Part model, mm, in its own coordinate system. A direction names the side the tool comes from. Round coordinates to 2 decimals unless told otherwise and drop trailing zeros. Loops run counter-clockwise (first coordinate to the right, second up) from the corner with the lowest first, then second, coordinate; pieces in that order, holes last.
(1) Tool access for faces 1 (the face through (48.6, 100.5, -4)), 2 (the face through (49, 79.5, 1)), 3 (the face through (48.56, 97.91, -5.65)): list every direction of +Z, -Z, +X, -X, +Y, -Y with a clear straight run to the whole face (end or side of a thin tool).
(2) Cut at A-A on x = 22. List the corners of the cut face in (y, z).
(3) Mould opens along Z. For faces 4 (the face through (98.5, 62, 0.3)), 5 (the face through (48.56, 97.3, -17.24)), 6 (the face through (49, 27, 3)) say: +Z half, -Z half, draft (parallel to the pull), parting line (faces both ways), or undercut.
(4) Cut at D-D on y = 38.5. List the corners of the cut face in (x, z).
(5) Flat gauge pins, fed straight in: pin 1 (10 mm diameter, centred on x = 81, z = -21.5, fed in from -Y); pin 2 (5.5 mm diameter, centred on x = 93.9, y = 21.3, fed in from -Z); pin 3 (1.5 mm diameter, centred on x = 58, z = 1.5, fed in from +Y). Where does each tip first touch, or does it go through?
(6) Cut at C-C on x = 85.7. List the corners of the cut face in (y, z).
(7) Probe probe 1 along X at (y, z) = (86.3, 1.65); probe 2 along Y at (x, z) = (93.9, 0.95); probe 3 along Y at (x, z) = (85.7, 0.75). List the from-to ranges inside material, lowest first.
(8) Cut at B-B on y = 10.8. List the corners of the cut face in (x, z).
from build123d import *

# Parameters (mm, degrees)
SKETCH1_W           = 98.5
SKETCH1_H           = 93.5
SKETCH1_W_2         = 78.5
SKETCH1_H_2         = 51.5
BOSS_EXTRUDE1_DEPTH = 3
CUT_EXTRUDE1_REACH  = 5
SKETCH2_R           = 3.5
SKETCH2_R_2         = 1.75
BOSS_EXTRUDE4_DEPTH = 98.5
BOSS_EXTRUDE5_DEPTH = 98.5


with BuildPart() as part:
    # Sketch1 → Boss-Extrude1 (new body)
    with BuildSketch(Plane.XY):
        with Locations((49.25, 46.75)):
            Rectangle(SKETCH1_W, SKETCH1_H)
        with Locations((49.25, 53.75)):
            Rectangle(SKETCH1_W_2, SKETCH1_H_2, mode=Mode.SUBTRACT)
    extrude(amount=BOSS_EXTRUDE1_DEPTH)

    # Sketch2 → Cut-Extrude1 (cut, up to next)
    with BuildSketch(Plane.XY.offset(3), mode=Mode.PRIVATE) as cut_extrude1_sk1:
        with Locations((85.7, 10.8)):
            Circle(SKETCH2_R)
    cut_extrude1_tool1 = extrude(cut_extrude1_sk1.sketch, amount=-CUT_EXTRUDE1_REACH, mode=Mode.PRIVATE) & part.part
    add(cut_extrude1_tool1.solids().sort_by_distance((85.7, 10.8, 3))[0], mode=Mode.SUBTRACT)
    # Sketch2 → Cut-Extrude1 (cut, up to next)
    with BuildSketch(Plane.XY.offset(3), mode=Mode.PRIVATE) as cut_extrude1_sk2:
        with Locations((93.9, 86.3)):
            Circle(SKETCH2_R_2)
    cut_extrude1_tool2 = extrude(cut_extrude1_sk2.sketch, amount=-CUT_EXTRUDE1_REACH, mode=Mode.PRIVATE) & part.part
    add(cut_extrude1_tool2.solids().sort_by_distance((93.9, 86.3, 3))[0], mode=Mode.SUBTRACT)
    # Sketch2 → Cut-Extrude1 (cut, up to next)
    with BuildSketch(Plane.XY.offset(3), mode=Mode.PRIVATE) as cut_extrude1_sk3:
        with Locations((93.9, 21.3)):
            Circle(SKETCH2_R_2)
    cut_extrude1_tool3 = extrude(cut_extrude1_sk3.sketch, amount=-CUT_EXTRUDE1_REACH, mode=Mode.PRIVATE) & part.part
    add(cut_extrude1_tool3.solids().sort_by_distance((93.9, 21.3, 3))[0], mode=Mode.SUBTRACT)
    # Sketch2 → Cut-Extrude1 (cut, up to next)
    with BuildSketch(Plane.XY.offset(3), mode=Mode.PRIVATE) as cut_extrude1_sk4:
        with Locations((6.3, 21.3)):
            Circle(SKETCH2_R_2)
    cut_extrude1_tool4 = extrude(cut_extrude1_sk4.sketch, amount=-CUT_EXTRUDE1_REACH, mode=Mode.PRIVATE) & part.part
    add(cut_extrude1_tool4.solids().sort_by_distance((6.3, 21.3, 3))[0], mode=Mode.SUBTRACT)
    # Sketch2 → Cut-Extrude1 (cut, up to next)
    with BuildSketch(Plane.XY.offset(3), mode=Mode.PRIVATE) as cut_extrude1_sk5:
        with Locations((6.3, 86.3)):
            Circle(SKETCH2_R_2)
    cut_extrude1_tool5 = extrude(cut_extrude1_sk5.sketch, amount=-CUT_EXTRUDE1_REACH, mode=Mode.PRIVATE) & part.part
    add(cut_extrude1_tool5.solids().sort_by_distance((6.3, 86.3, 3))[0], mode=Mode.SUBTRACT)

    # Sketch5 → Boss-Extrude4 (add)
    with BuildSketch(Plane.ZY):
        Polygon((3, 93.5), (-11.142135624, 107.642135624), (-13.263455967, 105.52081528), (0.878679656, 91.378679656), align=None)
    extrude(amount=-BOSS_EXTRUDE4_DEPTH)

    # Sketch6 → Boss-Extrude5 (add)
    with BuildSketch(Plane.ZY):
        Polygon((-11.142135624, 107.642135624), (-25.284271247, 93.5), (-23.162950904, 91.378679656), (-9.02081528, 105.52081528), align=None)
    extrude(amount=-BOSS_EXTRUDE5_DEPTH)


solid = part.part
Final values:
1. face 1: +Z, +X, -X, +Y
1. face 2: +Z, -Z
1. face 3: +X, -X, -Y
2. outline: (0, 0) - (28, 0) - (28, 3) - (0, 3) - close; (79.5, 0) - (92.26, 0) - (103.4, -11.14) - (91.38, -23.16) - (93.5, -25.28) - (107.64, -11.14) - (93.5, 3) - (79.5, 3) - close
3. face 4: draft
3. face 5: undercut
3. face 6: +Z half
4. outline: (0, 0) - (10, 0) - (10, 3) - (0, 3) - close; (88.5, 0) - (98.5, 0) - (98.5, 3) - (88.5, 3) - close
5. pin 1: stops at y = 91.38
5. pin 2: stops at z = 0
5. pin 3: stops at y = 95.75
6. outline: (0, 0) - (7.3, 0) - (7.3, 3) - (0, 3) - close; (14.3, 0) - (28, 0) - (28, 3) - (14.3, 3) - close; (79.5, 0) - (92.26, 0) - (103.4, -11.14) - (91.38, -23.16) - (93.5, -25.28) - (107.64, -11.14) - (93.5, 3) - (79.5, 3) - close
7. probe 1: x = 0 to 4.55, 8.05 to 92.15, 95.65 to 98.5
7. probe 2: y = 0 to 19.55, 23.05 to 84.55, 88.05 to 95.55
7. probe 3: y = 0 to 7.3, 14.3 to 28, 79.5 to 95.75
8. outline: (0, 0) - (82.2, 0) - (82.2, 3) - (0, 3) - close; (89.2, 0) - (98.5, 0) - (98.5, 3) - (89.2, 3) - close
